Check sheet for the modelled part. Datum: model origin and axes. Units: mm. Face numbers are marked on the shaded views. A direction names the side the tool comes from. Round coordinates to 2 decimals unless told otherwise and drop trailing zeros. Order: outer loops, then holes, each group sorted by start corner. A loop starts at its lowest first (then second) coordinate and runs counter-clockwise, first axis right, second up.
Q1. Scan lines: probe 1 along Z at (x, y) = (-16, -374); probe 2 along Z at (x, y) = (47, -547); probe 3 along Y at (x, z) = (37.5, -181.5). Record each from-to range of solid material in increasing order.
Q2. Depth check by flat-ended pin: P1, Ø1.5, axis at y = -92.5, z = 32.5, coming from the +X side; P2, Ø3, axis at x = -31.5, z = -194, coming from the +Y side; P3, Ø6, axis at x = 179, z = -1, coming from the -Y side. Enter the tip coordinate at first touch or a pass-through.
Q3. Cross-section at B-B on y = -352.5. Record the cut outline in (x, z).
Q4. Mould release check, pull along Z, two halves, no side actions. Record for the marked faces 1, 2, 3 and 4: +Z half, -Z half, draft (parallel to the pull), parting line (faces both ways), or undercut.
Q5. Cross-section at C-C on z = -93.5. Record the cut outline in (x, y).
Q6. Cross-section at D-D on x = 332.5. Record the cut outline in (y, z), then the cut area to 3 significant figures.
Q7. Set-up check for the marked faces 5, 6, 7 and 8: record each of +Z, -Z, +X, -X, +Y, -Y from which the full face is reachable in a straight line by a thin tool's end or side.
Q8. Cross-section at A-A on x = -62.5. Record the cut outline in (y, z), then the cut area to 3 significant figures.
from build123d import *

# Parameters (mm, degrees)
F0_W      = 540
F0_H      = 380
F0_W_2    = 440
F0_H_2    = 280
F1_DEPTH  = 560
F2_W      = 490
F2_H      = 500
F3_DEPTH  = 10
F4_W      = 700
F4_H      = 700
F5_DEPTH  = 50
F6_W      = 440
F6_H      = 280
F7_DEPTH  = 6
F8_W      = 440
F8_H      = 55
F9_DEPTH  = 480
F10_W     = 440
F10_H     = 300
F11_DEPTH = 40


with BuildPart() as f1:
    # F0 (on Front) → F1 (new body)
    with BuildSketch(Plane.XZ):
        Rectangle(F0_W, F0_H)
        Rectangle(F0_W_2, F0_H_2, mode=Mode.SUBTRACT)
    extrude(amount=F1_DEPTH)

    # F2 (on face) → F3 (join)
    with BuildSketch(Plane(origin=(0, 0, -190), x_dir=(1, 0, 0), z_dir=(0, 0, -1))):
        with Locations((25, 280)):
            Rectangle(F2_W, F2_H)
    extrude(amount=F3_DEPTH)

    # F4 (on face) → F5 (join)
    with BuildSketch(Plane(origin=(0, 0, -200), x_dir=(1, 0, 0), z_dir=(0, 0, -1))):
        with Locations((80, 280)):
            Rectangle(F4_W, F4_H)
    extrude(amount=F5_DEPTH)

    # F6 (on face) → F7 (join)
    with BuildSketch(Plane(origin=(0, 0, 0), x_dir=(-1, 0, 0), z_dir=(0, 1, 0))):
        Rectangle(F6_W, F6_H)
    extrude(amount=-F7_DEPTH)

    # F8 (on face) → F9 (cut)
    with BuildSketch(Plane.YZ.offset(270)):
        with Locations((-280, -172.5)):
            Rectangle(F8_W, F8_H)
    extrude(amount=-F9_DEPTH, mode=Mode.SUBTRACT)

    # F10 (on face) → F11 (cut)
    with BuildSketch(Plane.YZ.offset(270)):
        with Locations((-280, 5)):
            Rectangle(F10_W, F10_H)
    extrude(amount=-F11_DEPTH, mode=Mode.SUBTRACT)


solid = f1.part
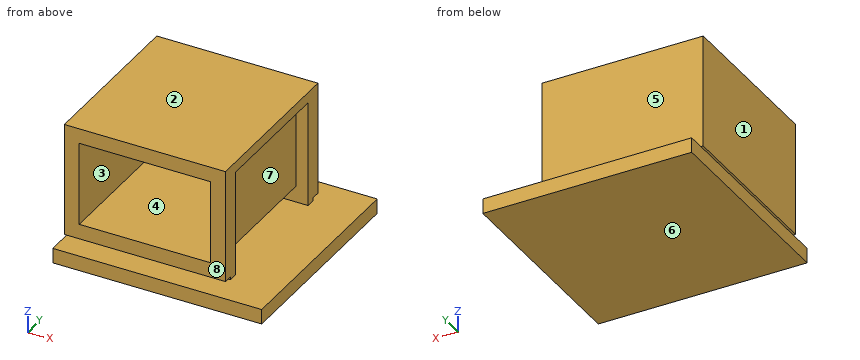
Results found:
1. probe 1: z = -250 to -200, -145 to -140, 140 to 190
1. probe 2: z = -250 to -200, -190 to -140, 140 to 190
1. probe 3: y = -560 to -500, -60 to 0
2. P1: stops at x = 230
2. P2: stops at y = -30
2. P3: stops at y = -6
3. outline: (-270, -250) - (430, -250) - (430, -200) - (-210, -200) - (-210, -145) - (230, -145) - (230, 155) - (270, 155) - (270, 190) - (-270, 190) - (-270, -190) - (-220, -190) - (-220, -200) - (-270, -200) - close; hole (-220, -140) - (220, -140) - (220, 140) - (-220, 140) - close
4. face 1: draft
4. face 2: +Z half
4. face 3: undercut
4. face 4: undercut
5. outline: (-270, -560) - (-220, -560) - (-220, -6) - (220, -6) - (220, -560) - (270, -560) - (270, -500) - (230, -500) - (230, -60) - (270, -60) - (270, 0) - (-270, 0) - close
6. outline: (-630, -250) - (70, -250) - (70, -200) - (-630, -200) - close
6. area: 35,000 mm2
7. face 5: +Z, +X, -X, +Y
7. face 6: -Z, +X, -X, +Y, -Y
7. face 7: +X
7. face 8: +Z, +X, -X, -Y
8. outline: (-630, -250) - (70, -250) - (70, -200) - (-30, -200) - (-30, -190) - (0, -190) - (0, 190) - (-560, 190) - (-560, 140) - (-6, 140) - (-6, -140) - (-560, -140) - (-560, -190) - (-530, -190) - (-530, -200) - (-630, -200) - close; hole (-500, -200) - (-60, -200) - (-60, -145) - (-500, -145) - close
8. area: 73,500 mm2
